Geometry check sheet. Reference: the model listing, model coordinates, mm. A direction names the side the tool comes from. Round coordinates to 2 decimals unless told otherwise and drop trailing zeros. Write each loop counter-clockwise with the first axis right and the second up, starting at its lowest first coordinate (ties: lowest second). Pieces come first, ordered by that corner, then holes. Notation, with made-up numbers: M 35,-16.75 L 40,-16.75 A23 cw 40,15.25 Z; hole C 48.25,6 d11. An arc over 180 degrees is marked long. Put each result on its own line as item: value. Start each with the question number.
(1) Gauge pin test, flat end, axial feed: pin 1 (1.5 mm diameter, centred on x = 31.5, y = -10.5, fed in from +Z). Record the tip position at first contact, or that the pin passes through.
(2) Mould release check, pull along X, two halves, no side actions. Record for faces 1 (the flat face through (120.5, -1, 14)), 2 (the flat face through (-120.5, -1, 14)), 3 (the flat face through (-136.5, -1, 8)), 4 (the flat face through (-2, 106.5, 8)): pulls with the +X half, pulls with the -X half, needs draft (parallel to the pull), parting line crosses it, or undercut.
(3) Material ranges on probe 1 along Y at (x, z) = (-103.5, 5); probe 2 along Y at (x, z) = (-8.5, 16.25); probe 3 along X at (y, z) = (-21.5, 12.5), recorded low to high.
(4) Section check B-B on z = 14. Record the cut outline in (x, y).
(5) Tool access check on faces 5 (the flat face through (-2, 1, 0)), 6 (the flat face through (-2, 1, 11)). Record the directions out of +Z, -Z, +X, -X, +Y, -Y that give a thin tool (end or side, any length) a straight path to the whole face; none if there is none.
(6) Section check A-A on y = 0. Record the cut outline in (x, z), then the cut area to 4 significant figures.
(7) Section check D-D on y = -63. Record the cut outline in (x, z).
(8) Section check C-C on x = -103.5. Record the cut outline in (y, z), then the cut area to 4 significant figures.
from build123d import *

# Parameters (mm, degrees)
F0_W     = 273
F0_H     = 213
F0_W_2   = 241
F0_H_2   = 181
F1_DEPTH = 17
F0_R     = 5
F2_DEPTH = 11


with BuildPart() as f1:
    # F0 (on Top) → F1 (new body)
    with BuildSketch(Plane.XY):
        Rectangle(F0_W, F0_H)
        Rectangle(F0_W_2, F0_H_2, mode=Mode.SUBTRACT)
    extrude(amount=F1_DEPTH)

    # F0 (on Top) → F2 (join)
    with BuildSketch(Plane.XY):
        Rectangle(F0_W_2, F0_H_2)
        with Locations((-103.5, 0)):
            Circle(F0_R, mode=Mode.SUBTRACT)
        with Locations((0, 73.5)):
            Circle(F0_R, mode=Mode.SUBTRACT)
    extrude(amount=F2_DEPTH)


solid = f1.part
Answers follow:
1. pin 1: stops at z = 11
2. face 1: undercut
2. face 2: undercut
2. face 3: pulls with the -X half
2. face 4: needs draft
3. probe 1: y = -106.5 to -5, 5 to 106.5
3. probe 2: y = -106.5 to -90.5, 90.5 to 106.5
3. probe 3: x = -136.5 to -120.5, 120.5 to 136.5
4. outline: M -136.5,-106.5 L 136.5,-106.5 L 136.5,106.5 L -136.5,106.5 Z; hole M -120.5,-90.5 L 120.5,-90.5 L 120.5,90.5 L -120.5,90.5 Z
5. face 5: -Z, +X, -X, +Y, -Y
5. face 6: +Z
6. outline: M -136.5,0 L -108.5,0 L -108.5,11 L -120.5,11 L -120.5,17 L -136.5,17 Z; M -98.5,0 L 136.5,0 L 136.5,17 L 120.5,17 L 120.5,11 L -98.5,11 Z
6. area: 3,085 mm^2
7. outline: M -136.5,0 L 136.5,0 L 136.5,17 L 120.5,17 L 120.5,11 L -120.5,11 L -120.5,17 L -136.5,17 Z
8. outline: M -106.5,0 L -5,0 L -5,11 L -90.5,11 L -90.5,17 L -106.5,17 Z; M 5,0 L 106.5,0 L 106.5,17 L 90.5,17 L 90.5,11 L 5,11 Z
8. area: 2,425 mm^2
